from build123d import *

# Parameters (mm, degrees)
RESSALTO_EXTRUS_O1_DEPTH = 54
CORTE_EXTRUS_O1_START    = 10
ESBO_O2_R                = 2
CORTE_EXTRUS_O1_DEPTH    = 14


with BuildPart() as part:
    # Esboço1 → Ressalto-extrusão1 (new body)
    with BuildSketch(Plane.XY):
        Polygon((0, 0), (16.52, 0), (16.52, 16.52), (15.32, 16.52), (15.32, 1.2), (0, 1.2), align=None)
    extrude(amount=RESSALTO_EXTRUS_O1_DEPTH)

    # Esboço2 → Corte-extrusão1 (cut)
    with BuildSketch(Plane(origin=(0, 0, 0), x_dir=(0, 0, -1), z_dir=(1, 0, 0)).offset(CORTE_EXTRUS_O1_START)):
        with Locations(Location((-5.2, 8.86, 0), (0, 0, 180))):
            Circle(ESBO_O2_R)
        with Locations(Location((-48.8, 8.86, 0), (0, 0, 180))):
            Circle(ESBO_O2_R)
    extrude(amount=CORTE_EXTRUS_O1_DEPTH, mode=Mode.SUBTRACT)


solid = part.part
Can you work these out from the model? Positions are in its coordinate system, mm. A direction names the side the tool comes from. Round coordinates to 2 decimals unless told otherwise and drop trailing zeros. Order: outer loops, then holes, each group sorted by start corner. A loop starts at its lowest first (then second) coordinate and runs counter-clockwise, first axis right, second up. Notation, with made-up numbers: M 5,-32.5 L 51,-32.5 A26 cw 51,-16.5 Z; hole C 2.25,68 d8. An arc over 180 degrees is marked long. Use a Markdown table: item, result.
1) On a 3-axis mill with a long thin cutter (end or side, diameter ignored), from which of +Z, -Z, +X, -X, +Y, -Y can I reach the whole of each face in a straight line? I mean faces 1 (the face through (15.912, 9.626, 7.047)), 2 (the face through (15.32, 9, 27)). Say none if no direction works.
Geometry says:
| item | result |
|---|---|
| face 1 | +X, -X |
| face 2 | +Z, -Z, -X, +Y |
2) Imagine slicing it at A-A (y = 8.86). List the corners of the cut face in (x, z) for me, then the cut area to 3 significant figures.
Geometry says:
| item | result |
|---|---|
| outline | M 15.32,0 L 16.52,0 L 16.52,3.2 L 15.32,3.2 Z; M 15.32,7.2 L 16.52,7.2 L 16.52,46.8 L 15.32,46.8 Z; M 15.32,50.8 L 16.52,50.8 L 16.52,54 L 15.32,54 Z |
| area | 55.2 mm² |
3) I'm going to push flat-ended pins straight in: P1, Ø5, axis at x = 7.5, y = 5, coming from the +Z side (1 decimal); P2, Ø4, axis at x = 13.5, z = 32, coming from the +Y side; P3, Ø8, axis at y = 14.5, z = 10.5, coming from the -X side. Where does each tip first touch, or does it pass through?
Geometry says:
| item | result |
|---|---|
| P1 | passes through |
| P2 | stops at y = 16.52 |
| P3 | stops at x = 15.32 |
4) Imagine slicing it at C-C (z = 41). List the corners of the cut face in (x, y) for me, then the cut area to 3 significant figures.
Geometry says:
| item | result |
|---|---|
| outline | M 0,0 L 16.52,0 L 16.52,16.52 L 15.32,16.52 L 15.32,1.2 L 0,1.2 Z |
| area | 38.2 mm² |
5) If we mould it in two halves opening along Z, with no side actions, what happens to faces 3 (the face through (16, 16.52, 27)), 4 (the face through (15.912, 9.626, 50.647)), 5 (the face through (12, 1, 0))? For each: +Z half, -Z half, draft (parallel to the pull), parting line (faces both ways), or undercut.
Geometry says:
| item | result |
|---|---|
| face 3 | draft |
| face 4 | undercut |
| face 5 | -Z half |
6) If I drill on line 1 along Y through (x, z) = (16.15, 48.8); line 2 along X through (y, z) = (11, 24.5); line 3 along Y through (x, z) = (6.5, 45), over which ranges is the centre line in solid material (lowest first)?
Geometry says:
| item | result |
|---|---|
| line 1 | y = 0 to 6.86, 10.86 to 16.52 |
| line 2 | x = 15.32 to 16.52 |
| line 3 | y = 0 to 1.2 |
7) Imagine slicing it at B-B (z = 48.8). List the corners of the cut face in (x, y) for me.
Geometry says:
| item | result |
|---|---|
| outline | M 0,0 L 16.52,0 L 16.52,6.86 L 15.32,6.86 L 15.32,1.2 L 0,1.2 Z; M 15.32,10.86 L 16.52,10.86 L 16.52,16.52 L 15.32,16.52 Z |
8) Imagine slicing it at D-D (y = 14.75). List the corners of the cut face in (x, z) for me, then the cut area to 3 significant figures.
Geometry says:
| item | result |
|---|---|
| outline | M 15.32,0 L 16.52,0 L 16.52,54 L 15.32,54 Z |
| area | 64.8 mm² |
